from build123d import *

# Parameters (mm, degrees)
F1_DEPTH = 38.1
F2_R     = 12.7
F3_R     = 4.365625
F4_DEPTH = 27.2490523559
F5_W     = 6.35
F5_H     = 38.1
F6_DEPTH = 6.35


with BuildPart() as f1:
    # F0 (on Front) → F1 (new body)
    with BuildSketch(Plane.XZ):
        with BuildLine():
            Line((0, 114.3), (0, 0))
            Line((0, 0), (203.2, 0))
            Line((203.2, 0), (203.2, 61.4492737428))
            ThreePointArc((203.2, 61.4492737428), (195.6130610643, 88.1564142385), (175.1184506514, 106.8861750456))
            Line((175.1184506514, 106.8861750456), (92.1354487885, 148.3776759771))
            ThreePointArc((92.1354487885, 148.3776759771), (83.8501970728, 151.3807864987), (75.0966107999, 152.4))
            Line((75.0966107999, 152.4), (38.1, 152.4))
            ThreePointArc((38.1, 152.4), (11.1592316368, 141.2407683632), (0, 114.3))
        make_face()
        with BuildLine():
            ThreePointArc((28.575, 101.6), (39.1156260332, 120.5057142156), (60.73932216, 121.47864432))
            Line((60.73932216, 121.47864432), (162.33932216, 70.67864432))
            ThreePointArc((162.33932216, 70.67864432), (174.100727981, 46.0011428347), (153.0305820147, 28.5839474406))
            Line((153.0305820147, 28.5839474406), (67.7559977395, 26.1635075802))
            ThreePointArc((67.7559977395, 26.1635075802), (40.119172145, 36.9278834801), (28.575, 64.2481691106))
            Line((28.575, 64.2481691106), (28.575, 101.6))
        make_face(mode=Mode.SUBTRACT)
    extrude(amount=F1_DEPTH)

    # F2
    f2_edges = [f1.edges().sort_by_distance(p)[0] for p in [
        (56.598305, -38.1, 152.4),
        (111.539322, -38.1, 96.078644),
        (111.539322, 0, 96.078644),
        (133.62695, 0, 127.631926),
    ]]
    fillet(f2_edges, radius=F2_R)

    # F3 (on face) → F4 (cut, through all)
    with BuildSketch(Plane(origin=(0, 0, 0), x_dir=(1, 0, 0), z_dir=(0, 0, -1))):
        with Locations((101.6, 19.05)):
            Circle(F3_R)
    extrude(amount=-F4_DEPTH, mode=Mode.SUBTRACT)

    # F5 (on face) → F6 (join)
    with BuildSketch(Plane(origin=(0, 0, 0), x_dir=(1, 0, 0), z_dir=(0, 0, -1))):
        with Locations((53.975, 19.05)):
            Rectangle(F5_W, F5_H)
        with Locations((149.225, 19.05)):
            Rectangle(F5_W, F5_H)
    extrude(amount=F6_DEPTH)


solid = f1.part
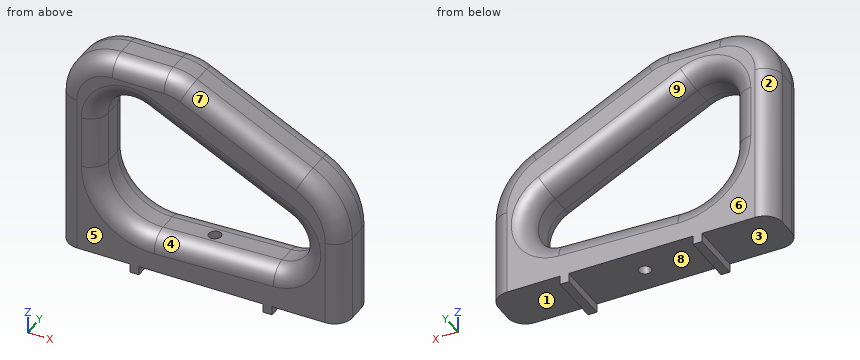
For this review, take the finished solid that the model builds, in its own axes (mm). Face numbers are marked on the shaded views. A direction names the side the tool comes from. Coordinates: 2 decimals unless noted, no trailing zeros. Order: outer loops, then holes, each group sorted by start corner. A loop starts at its lowest first (then second) coordinate and runs counter-clockwise, first axis right, second up. Notation, with made-up numbers: (2, 50.25) -> (32, 50.25) arc R20 ccw to (32, 70.25) -> close; hole circle Ø5 at (-19.75, 78). An arc over 180 degrees is marked (long way). Return JSON: item names as keys, results as strings.
1. Machinability: for the marked faces 1, 2, 3, 4 and 5, which of the approach directions +Z, -Z, +X, -X, +Y, -Y give a long, thin tool a straight path to every point of the face, cutting with its end or side? Answer none if there is none.
Answer block:
{"face 1": "-Z, +X, +Y, -Y", "face 2": "+Z, -Z, -X, +Y", "face 3": "-Z, -X, +Y, -Y", "face 4": "-Y", "face 5": "+Z, -Z, +X, -X, -Y"}
2. We need section C-C on x = 101.6. State how many separate pieces and enclosed holes the cut face has, and give its area (3 significant figures).
Answer block:
{"separate pieces": "3", "enclosed holes": "0", "area": "2,200 mm²"}
3. We need section A-A on z = 11. Write out the cut boundary in (x, y), and give its area (3 significant figures).
Answer block:
{"outline": "(0, -25.4) arc R12.7 ccw to (12.7, -38.1) -> (190.5, -38.1) arc R12.7 ccw to (203.2, -25.4) -> (203.2, -12.7) arc R12.7 ccw to (190.5, 0) -> (12.7, 0) arc R12.7 ccw to (0, -12.7) -> close; hole circle Ø8.73 at (101.6, -19.05)", "area": "7,540 mm²"}
4. For line 1 (X direction, y = -19, z = 8); line 2 (Y direction, x = 101.6, z = 12.25); line 3 (Z direction, x = 116, y = -9), list the stretches that pass through material, from the lowest coordinate up. Write a range as from..to.
Answer block:
{"line 1": "0..97.23, 105.97..203.2", "line 2": "-38.1..-23.42, -14.68..0", "line 3": "0..26.98, 94.46..135.83"}
5. For pin 1 Ø3 at (y, z) = (-12, -2.5) entering from +X; pin 2 Ø11.5 at (x, y) = (101.6, -19.05) entering from -Z; pin 3 Ø3 at (x, z) = (151, 117) entering from -Y, all flat-tipped, find the tip position at first contact; note any pin that passes through.
Answer block:
{"pin 1": "x = 152.4", "pin 2": "z = 0", "pin 3": "y = -33.87"}
6. The part is to be moulded in two halves that separate along Z. For the marked faces 6, 7, 8 and 9, say which applies: +Z half, -Z half, draft (parallel to the pull), parting line (faces both ways), or undercut.
Answer block:
{"face 6": "draft", "face 7": "+Z half", "face 8": "-Z half", "face 9": "undercut"}
